Can you work these out from the model? Positions are in its coordinate system, mm. Face numbers are marked on the shaded views. A direction names the side the tool comes from. Give positions to 0.01 mm unless a question says otherwise; leave off trailing zeros. Write each loop counter-clockwise with the first axis right and the second up, starting at its lowest first coordinate (ties: lowest second). Pieces come first, ordered by that corner, then holes.
from build123d import *

# Parameters (mm, degrees)
ESQUISSE1_R        = 10
BOSS_EXTRU_1_DEPTH = 62
ESQUISSE2_R        = 8
BOSS_EXTRU_2_DEPTH = 5
ESQUISSE3_R        = 5
BOSS_EXTRU_3_DEPTH = 14


with BuildPart() as part:
    # Esquisse1 → Boss.-Extru.1 (new body)
    with BuildSketch(Plane(origin=(0, 0, 0), x_dir=(1, 0, 0), z_dir=(0, 1, 0))):
        with Locations(Location((0, 0, 0), (0, 0, 270))):  # turned: the seam where the file's is
            Circle(ESQUISSE1_R)
    extrude(amount=BOSS_EXTRU_1_DEPTH)

    # Esquisse2 → Boss.-Extru.2 (add)
    with BuildSketch(Plane(origin=(0, 62, 0), x_dir=(1, 0, 0), z_dir=(0, 1, 0))):
        with Locations(Location((0, 0, 0), (0, 0, 270))):  # turned: the seam where the file's is
            Circle(ESQUISSE2_R)
    extrude(amount=BOSS_EXTRU_2_DEPTH)

    # Esquisse3 → Boss.-Extru.3 (add)
    with BuildSketch(Plane(origin=(0, 67, 0), x_dir=(1, 0, 0), z_dir=(0, 1, 0))):
        with Locations(Location((0, 0, 0), (0, 0, 270))):  # turned: the seam where the file's is
            Circle(ESQUISSE3_R)
    extrude(amount=BOSS_EXTRU_3_DEPTH)


solid = part.part
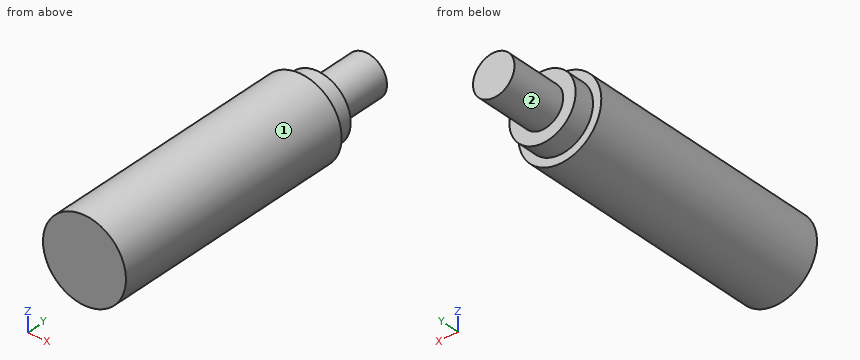
(1) If I drill on L1, parallel to Z at x = 6, y = 52.5; L2, parallel to Y at x = -6.75, z = 0.25; L3, parallel to Y at x = -6, z = 5.5, over which ranges is the centre line in solid material (lowest first)?
Returned:
L1: z = -8 to 8
L2: y = 0 to 67
L3: y = 0 to 62
(2) Imagine slicing it at A-A, the plane z = 0. Write out the boundary of the cut face in (x, y), plus the area to 3 significant figures.
Returned:
outline: (-10, 0) - (10, 0) - (10, 62) - (8, 62) - (8, 67) - (5, 67) - (5, 81) - (-5, 81) - (-5, 67) - (-8, 67) - (-8, 62) - (-10, 62) - close
area: 1,460 mm2
(3) Imagine slicing it at C-C, the plane y = 42.5. Write out the boundary of the cut face in (x, z).
Returned:
outline: circle Ø20 at (0, 0)
(4) For the marked faces 1 and 2, which set-ups out of +Z, -Z, +X, -X, +Y, -Y let a thin tool reach every point of the face, with its end or its side?
Returned:
face 1: +Y, -Y
face 2: +Y
(5) Imagine slicing it at D-D, the plane z = -6.5. Write out the boundary of the cut face in (x, y).
Returned:
outline: (-7.6, 0) - (7.6, 0) - (7.6, 62) - (4.66, 62) - (4.66, 67) - (-4.66, 67) - (-4.66, 62) - (-7.6, 62) - close
(6) Imagine slicing it at B-B, the plane x = 0. Write out the boundary of the cut face in (y, z).
Returned:
outline: (0, -10) - (62, -10) - (62, -8) - (67, -8) - (67, -5) - (81, -5) - (81, 5) - (67, 5) - (67, 8) - (62, 8) - (62, 10) - (0, 10) - close
(7) Will this pin go through, and if not, where does the flat tip stop? P1, Ø1, axis at y = 70, z = 2.5, coming from the -X side.
Returned:
P1: stops at x = -4.58
